```python
from build123d import *

# Parameters (mm, degrees)
BOSS_EXTRUDE1_DEPTH   = 3.000000096
BOSS_EXTRUDE2_DEPTH   = 2.206999904
SKETCH2_R             = 3.175
CUT_EXTRUDE1_DEPTH    = 6.207
SKETCH3_W             = 2.54
SKETCH3_H             = 0.635
SKETCH3_W_2           = 0.635
SKETCH3_H_2           = 2.54
SKETCH3_W_3           = 12.723081303
SKETCH3_H_3           = 1.613636956
CUT_EXTRUDE2_DEPTH    = 6.207
F_6_32_TAPPED_HOLE1_D = 2.7051


with BuildPart() as part:
    # Sketch1 → Boss-Extrude1 (new body)
    with BuildSketch(Plane.XY):
        with BuildLine():
            Line((8.696654013, 17.676910134), (44.336045576, 53.316301697))
            ThreePointArc((44.336045576, 53.316301697), (26.536034567, 64.063654543), (6.35, 69.050636956))
            Line((6.35, 69.050636956), (6.35, 18.648926052))
            Line((6.35, 18.648926052), (4.88230096, 15.105587123))
            ThreePointArc((4.88230096, 15.105587123), (-6.075099489, 14.666587579), (-14.133571205, 7.228954972))
            Line((-14.133571205, 7.228954972), (-17.676910134, 8.696654013))
            Line((-17.676910134, 8.696654013), (-76.191723231, 67.21146711))
            ThreePointArc((-76.191723231, 67.21146711), (-38.880636728, 93.866160503), (6.35, 101.401368334))
            Line((6.35, 101.401368334), (6.35, 81.795887818))
            ThreePointArc((6.35, 81.795887818), (31.396114158, 75.796924606), (53.348298889, 62.32855501))
            Line((53.348298889, 62.32855501), (67.21146711, 76.191723231))
            ThreePointArc((67.21146711, 76.191723231), (93.866160503, 38.880636728), (101.401368334, -6.35))
            Line((101.401368334, -6.35), (18.648926052, -6.35))
            Line((18.648926052, -6.35), (15.105587123, -4.88230096))
            ThreePointArc((15.105587123, -4.88230096), (14.666587579, 6.075099489), (7.228954972, 14.133571205))
            Line((7.228954972, 14.133571205), (8.696654013, 17.676910134))
        make_face()
        with BuildLine():
            Line((88.672924278, 6.35), (27.86051193, 6.35))
            ThreePointArc((27.86051193, 6.35), (26.399857642, 10.93517908), (24.190484974, 15.210228852))
            Line((24.190484974, 15.210228852), (67.191354125, 58.211098004))
            ThreePointArc((67.191354125, 58.211098004), (82.13289044, 34.020557137), (88.672924278, 6.35))
        make_face(mode=Mode.SUBTRACT)
        with BuildLine():
            Line((-58.211098004, 67.191354125), (-15.210228852, 24.190484974))
            ThreePointArc((-15.210228852, 24.190484974), (-10.93517908, 26.399857642), (-6.35, 27.86051193))
            Line((-6.35, 27.86051193), (-6.35, 88.672924278))
            ThreePointArc((-6.35, 88.672924278), (-34.020557137, 82.13289044), (-58.211098004, 67.191354125))
        make_face(mode=Mode.SUBTRACT)
    extrude(amount=BOSS_EXTRUDE1_DEPTH)

    # Sketch4 → Boss-Extrude2 (add)
    with BuildSketch(Plane(origin=(0, 0, 0), x_dir=(-1, 0, 0), z_dir=(0, 0, -1))):
        with BuildLine():
            Line((67.191354125, 58.211098004), (76.191723231, 67.21146711))
            ThreePointArc((76.191723231, 67.21146711), (38.880636728, 93.866160503), (-6.35, 101.401368334))
            Line((-6.35, 101.401368334), (-6.35, 88.672924278))
            ThreePointArc((-6.35, 88.672924278), (34.020557137, 82.13289044), (67.191354125, 58.211098004))
        make_face()
        with BuildLine():
            Line((-58.211098004, 67.191354125), (-67.21146711, 76.191723231))
            ThreePointArc((-67.21146711, 76.191723231), (-93.866160503, 38.880636728), (-101.401368334, -6.35))
            Line((-101.401368334, -6.35), (-88.672924278, -6.35))
            ThreePointArc((-88.672924278, -6.35), (-82.13289044, 34.020557137), (-58.211098004, 67.191354125))
        make_face()
    extrude(amount=BOSS_EXTRUDE2_DEPTH)

    # Sketch2 → Cut-Extrude1 (cut, through all)
    with BuildSketch(Plane.XY.offset(3.000000096)):
        with Locations((22.225, 0)):
            Circle(SKETCH2_R)
        with Locations((36.195, 0)):
            Circle(SKETCH2_R)
        with Locations((61.722, 0)):
            Circle(SKETCH2_R)
        with Locations((75.692, 0)):
            Circle(SKETCH2_R)
        with Locations((53.522326482, 53.522326482)):
            Circle(SKETCH2_R)
        with Locations((43.644044748, 43.644044748)):
            Circle(SKETCH2_R)
        with Locations((25.593729945, 25.593729945)):
            Circle(SKETCH2_R)
        with Locations((15.715448212, 15.715448212)):
            Circle(SKETCH2_R)
        with Locations((0, 75.692)):
            Circle(SKETCH2_R)
        with Locations((0, 61.722)):
            Circle(SKETCH2_R)
        with Locations((0, 36.195)):
            Circle(SKETCH2_R)
        with Locations((0, 22.225)):
            Circle(SKETCH2_R)
        with Locations((-53.522326482, 53.522326482)):
            Circle(SKETCH2_R)
        with Locations((-43.644044748, 43.644044748)):
            Circle(SKETCH2_R)
        with Locations((-25.593729945, 25.593729945)):
            Circle(SKETCH2_R)
        with Locations((-15.715448212, 15.715448212)):
            Circle(SKETCH2_R)
    extrude(amount=-CUT_EXTRUDE1_DEPTH, mode=Mode.SUBTRACT)

    # Sketch3 → Cut-Extrude2 (cut, through all)
    with BuildSketch(Plane.XY.offset(3.000000096)):
        Polygon((15.266435406, 24.246691527), (17.06248663, 26.042742751), (17.511499436, 25.593729945), (15.715448212, 23.797678721), align=None)
        Polygon((55.048970022, 64.029226143), (56.845021246, 65.825277367), (65.85268206, 56.817616554), (64.056630836, 55.02156533), align=None)
        Polygon((29.230733674, 38.210989795), (31.026784898, 40.007041019), (31.475797704, 39.558028213), (29.67974648, 37.761976989), align=None)
        with Locations((29.21, -6.0325)):
            Rectangle(SKETCH3_W, SKETCH3_H)
        with Locations((68.707, -6.0325)):
            Rectangle(SKETCH3_W, SKETCH3_H)
        Polygon((-65.825277367, 56.845021246), (-64.029226143, 55.048970022), (-63.580213337, 55.497982828), (-65.376264561, 57.294034052), align=None)
        Polygon((43.195031942, 52.175288063), (44.336045576, 53.316301697), (44.785058382, 52.867288891), (43.644044748, 51.726275257), align=None)
        with Locations((48.9585, -6.0325)):
            Rectangle(SKETCH3_W, SKETCH3_H)
        with Locations((85.471, -6.0325)):
            Rectangle(SKETCH3_W, SKETCH3_H)
        Polygon((99.935462164, 14.437711971), (100.266998693, 11.919442024), (101.526133667, 12.085210288), (101.194597138, 14.603480236), align=None)
        Polygon((93.765504959, 37.464305742), (94.938831965, 37.950313702), (93.966816047, 40.296967714), (92.793489041, 39.810959755), align=None)
        Polygon((79.327792988, 62.471156422), (80.874047017, 60.456038938), (81.88160576, 61.229165953), (80.33535173, 63.244283437), align=None)
        Polygon((13.593916116, 7.005422516), (14.565932035, 4.658768503), (15.739259041, 5.144776462), (14.767243123, 7.491430475), align=None)
        Polygon((-24.246691527, 15.266435406), (-26.042742751, 17.06248663), (-25.593729945, 17.511499436), (-23.797678721, 15.715448212), align=None)
        Polygon((-40.007041019, 31.026784898), (-38.210989795, 29.230733674), (-37.761976989, 29.67974648), (-39.558028213, 31.475797704), align=None)
        Polygon((-63.244283437, 80.33535173), (-61.229165953, 81.88160576), (-60.456038938, 80.874047017), (-62.471156422, 79.327792988), align=None)
        Polygon((-37.950313702, 94.938831965), (-40.296967714, 93.966816047), (-39.810959755, 92.793489041), (-37.464305742, 93.765504959), align=None)
        Polygon((-14.437711971, 99.935462164), (-14.603480236, 101.194597138), (-12.085210288, 101.526133667), (-11.919442024, 100.266998693), align=None)
        with Locations((6.0325, 85.471)):
            Rectangle(SKETCH3_W_2, SKETCH3_H_2)
        with Locations((6.0325, 48.9585)):
            Rectangle(SKETCH3_W_2, SKETCH3_H_2)
        with Locations((6.0325, 29.21)):
            Rectangle(SKETCH3_W_2, SKETCH3_H_2)
        Polygon((-7.491430475, 14.767243123), (-5.144776462, 15.739259041), (-4.658768503, 14.565932035), (-7.005422516, 13.593916116), align=None)
        with Locations((-0.011540651, 68.243818478)):
            Rectangle(SKETCH3_W_3, SKETCH3_H_3)
        Polygon((-53.971339288, 44.991083167), (-52.175288063, 43.195031942), (-51.726275257, 43.644044748), (-53.522326482, 45.440095973), align=None)
    extrude(amount=-CUT_EXTRUDE2_DEPTH, mode=Mode.SUBTRACT)

    # #6-32 Tapped Hole1 (through all)
    with Locations(Plane.XY.offset(3.000000096)):
        with Locations((95.25, 0), (92.004434954, 24.652514046), (82.48891971, 47.625), (67.351920908, 67.351920908), (47.625, 82.48891971), (24.652514046, 92.004434954), (0, 95.25), (-24.652514046, 92.004434954), (-47.625, 82.48891971), (-67.351920908, 67.351920908)):
            Hole(F_6_32_TAPPED_HOLE1_D / 2)


solid = part.part
```
Source: CAD feature listing. Evaluate the final solid. Frame: model axes, mm. A direction names the side the tool comes from. Round coordinates to 2 decimals unless told otherwise and drop trailing zeros.
1. Ray query, L1, parallel to X at y = 41, z = 1.75; L2, parallel to Y at x = -56, z = 1.45; L3, parallel to X at y = 42, z = 1.5. Return the intervals inside material, ascending.
2. Section query A-A on z = -0.95. Give the number of separate pieces and of enclosed holes in the cut face, and give its area (3 significant figures).
3. Mould query, pull axis X, two halves, no side actions, for faces 1 (the flat face through (23.06, 32.04, 1.48)), 2 (the flat face through (6.35, 94, 0)), 3 (the cylindrical face through (-50.95, 87.9, 0.43)). Classes: released by +X, released by -X, zero draft, split by the parting line, or undercut.
4. Access query for faces 4 (the flat face through (61.96, 70.94, 0.36)), 5 (the cylindrical face through (-11.18, 11.27, 1.48)), 6 (the cylindrical face through (26.81, 63.95, 1.48)). Directions: +Z, -Z, +X, -X, +Y, -Y. A direction counts if a zero-diameter tool reaches every point of the face in a straight line with its end or side. Return the directions, or none.
5. Contact query for flat-ended pins moving along their axis: pin 1 (1.3 mm diameter, centred on y = 49, z = 1.5, fed in from +X); pin 2 (2 mm diameter, centred on x = -24.65, y = 92, fed in from +Z); pin 3 (4.5 mm diameter, centred on x = 67.35, y = 67.35, fed in from +Z); pin 4 (1.9 mm diameter, centred on y = 83, z = 1, fed in from +X). Output: stop coordinate, or through.
Answers below:
1. L1: x = -49.98 to -45.4, -41.89 to -32.02, -6.35 to 6.35, 32.02 to 41.89, 45.4 to 49.98, 78.88 to 92.96
1. L2: y = 47.02 to 51.54, 55.51 to 64.98, 69.04 to 84.77
1. L3: x = -50.98 to -46.36, -40.93 to -33.02, -6.35 to 6.35, 33.02 to 40.93, 46.36 to 50.98, 78.35 to 92.51
2. separate pieces: 2
2. enclosed holes: 8
2. area: 2,170 mm2
3. face 1: undercut
3. face 2: released by +X
3. face 3: released by -X
4. face 4: +Z, -Z, +Y
4. face 5: +Z, -Z, -Y
4. face 6: +Z, -Z
5. pin 1: stops at x = 89.36
5. pin 2: passes through
5. pin 3: stops at z = 3
5. pin 4: stops at x = 6.35
